Build history of the part. All positions in model axes, mm. Face numbers are marked on the shaded views. Coordinates: 2 decimals unless noted, no trailing zeros. Order: outer loops, then holes, each group sorted by start corner. A loop starts at its lowest first (then second) coordinate and runs counter-clockwise, first axis right, second up. Notation, with made-up numbers: M 59.25,-24 L 101.25,-24 A31 cw 101.25,0 Z; hole C 33.5,40 d4. An arc over 180 degrees is marked long. Use a Markdown table: item, result. Add a question column.
from build123d import *

# Parameters (mm, degrees)
SKETCH_1_W       = 25
SKETCH_1_H       = 25
EXTRUDE_1_DEPTH  = 25
FILLET_1_R       = 3
CHAMFER_1_SIZE   = 3
FILLET_1_2_DEPTH = 25


with BuildPart() as part:
    # 草图1 → 凸台-拉伸1 (new body)
    with BuildSketch(Plane.XY):
        with Locations((12.5, 12.5)):
            Rectangle(SKETCH_1_W, SKETCH_1_H)
    extrude(amount=EXTRUDE_1_DEPTH)

    # 草图2 → 切除-旋转1 (revolve, cut)
    with BuildSketch(Plane.XY.offset(12.5), mode=Mode.PRIVATE) as cut_revolve_1_sk:
        Polygon((10.25, 0), (10.25, 23.35), (8.6, 25), (12.5, 25), (12.5, 0), align=None)
    revolve(cut_revolve_1_sk.sketch.rotate(Axis((12.5, 25, 12.5), (0, -1, 0)), 270), axis=Axis((12.5, 25, 12.5), (0, -1, 0)), mode=Mode.SUBTRACT)

    # Fillet 1
    fillet_1_edges = [part.edges().sort_by_distance(p)[0] for p in [
        (25, 12.5, 25),
        (12.5, 25, 25),
        (25, 12.5, 0),
        (25, 25, 12.5),
        (25, 0, 12.5),
    ]]
    fillet(fillet_1_edges, radius=FILLET_1_R)

    # 倒角1
    chamfer_1_edges = [part.edges().sort_by_distance(p)[0] for p in [
        (0, 11, 25),
        (0, 25, 11),
        (0, 24.121320344, 24.121320344),
        (0, 12.5, 0),
        (0, 0, 12.5),
    ]]
    chamfer(chamfer_1_edges, length=CHAMFER_1_SIZE)

    # Fillet 1 2: read off the stored shape, not the designer's step
    # Fillet 1 2 outline → Fillet 1 2 (cut)
    with BuildSketch(Plane(origin=(0, 0, 0), x_dir=(1, 0, 0), z_dir=(0, 1, 0))):
        with BuildLine():
            ThreePointArc((0, -4.656854249), (0.30448187, -3.12612052), (1.171572875, -1.828427125))
            Line((1.171572875, -1.828427125), (0, -3))
            Line((0, -3), (0, -4.656854249))
        make_face()
    extrude(amount=FILLET_1_2_DEPTH, mode=Mode.SUBTRACT)


solid = part.part
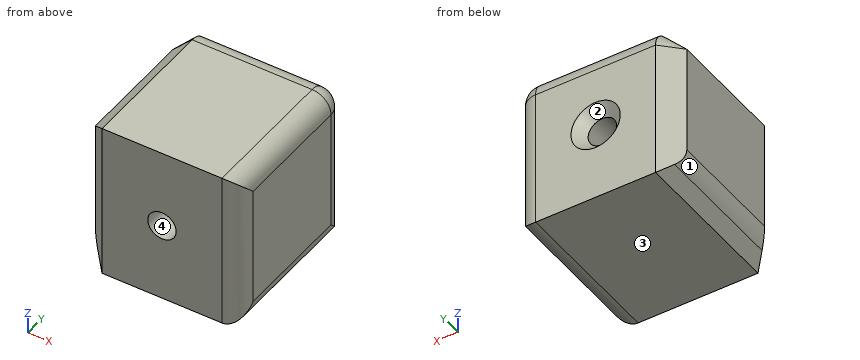
(1) Slice it at C-C on y = 15.5. Give the cut face in (x, z), and give its area (3 significant figures).
(2) Slice it at D-D on z = 18. Give the cut face in (x, y), and give its area (3 significant figures).
(3) Drill centre lines: line 1 along X through (y, z) = (12.75, 12.5); line 2 along Y through (x, z) = (2.75, 8.25). Where is each one in solid material? Low to high. Write a range as from..to.
(4) Slice it at B-B on x = 12.5. Give the cut face in (y, z).
(5) Slice it at A-A on z = 12.5. Give the cut face in (x, y), and give its area (3 significant figures).
(6) Mould opens along X. For the marked faces 1, 2, 3 and 4 say: released by +X, released by -X, zero draft, split by the parting line, or undercut.
Solutions:
| question | item | result |
|---|---|---|
| 1 | outline | M 0,4.66 A4 ccw 1.17,1.83 L 3,0 L 22,0 A3 ccw 25,3 L 25,22 A3 ccw 22,25 L 3,25 L 0,22 Z; hole C 12.5,12.5 d4.5 |
| 1 | area | 596 mm² |
| 2 | outline | M 0,3 L 3,0 L 22,0 A3 ccw 25,3 L 25,22 A3 ccw 22,25 L 3,25 L 0,22 Z |
| 2 | area | 612 mm² |
| 3 | line 1 | 0..10.25, 14.75..25 |
| 3 | line 2 | 0.25..24.75 |
| 4 | outline | M 0,0 L 25,0 L 25,8.6 L 23.35,10.25 L 0,10.25 Z; M 0,14.75 L 23.35,14.75 L 25,16.4 L 25,22 A3 ccw 22,25 L 0,25 Z |
| 5 | outline | M 0,3 L 3,0 L 10.25,0 L 10.25,23.35 L 8.6,25 L 3,25 L 0,22 Z; M 14.75,0 L 22,0 A3 ccw 25,3 L 25,22 A3 ccw 22,25 L 16.4,25 L 14.75,23.35 Z |
| 5 | area | 497 mm² |
| 6 | face 1 | released by -X |
| 6 | face 2 | undercut |
| 6 | face 3 | zero draft |
| 6 | face 4 | undercut |
